For this review, take the finished solid that the model builds, in its own axes (mm). A direction names the side the tool comes from. Give positions to 0.01 mm unless a question says otherwise; leave off trailing zeros. Loops run counter-clockwise (first coordinate to the right, second up) from the corner with the lowest first, then second, coordinate; pieces in that order, holes last. Notation, with made-up numbers: (35, 2.5) - (57, 2.5) arc R20 ccw to (57, 15.5) - close; hole circle Ø8 at (19.5, 72.5). An arc over 180 degrees is marked (long way). Answer in a Markdown table with one row per item.
```python
from build123d import *

# Parameters (mm, degrees)
SKETCH_2_W          = 57
SKETCH_2_H          = 40.4
EXTRUDE_1_DEPTH     = 1.5
SKETCH_4_R          = 3
SKETCH_4_R_2        = 1.5
EXTRUDE_3_DEPTH     = 4
SKETCH_5_W          = 57
SKETCH_5_H          = 4.2
CUT_EXTRUDE_1_DEPTH = 2.5
SKETCH_6_W          = 1
SKETCH_6_H          = 32
EXTRUDE_4_DEPTH     = 1.5
SKETCH_8_R          = 3
SKETCH_8_R_2        = 1.5
CUT_EXTRUDE_3_DEPTH = 2
SKETCH_7_R          = 1.5
CUT_EXTRUDE_4_DEPTH = 4.5


with BuildPart() as part:
    # 草图2 → 凸台-拉伸1 (new body)
    with BuildSketch(Plane(origin=(0, 0, 0), x_dir=(1, 0, 0), z_dir=(0, 1, 0))):
        with Locations((3.861898857, -4.534326193)):
            Rectangle(SKETCH_2_W, SKETCH_2_H)
    extrude(amount=EXTRUDE_1_DEPTH)

    # 草图4 → 凸台-拉伸3 (add)
    with BuildSketch(Plane(origin=(0, 1.5, 0), x_dir=(1, 0, 0), z_dir=(0, 1, 0))):
        with Locations((-22.099370277, 7.765673807)):
            Circle(SKETCH_4_R)
        with Locations((-22.099370277, 7.765673807)):
            Circle(SKETCH_4_R_2, mode=Mode.SUBTRACT)
        with Locations((-22.138101143, -16.834326193)):
            Circle(SKETCH_4_R)
        with Locations((-22.138101143, -16.834326193)):
            Circle(SKETCH_4_R_2, mode=Mode.SUBTRACT)
        with Locations((29.861898857, -16.834326193)):
            Circle(SKETCH_4_R)
        with Locations((29.861898857, -16.834326193)):
            Circle(SKETCH_4_R_2, mode=Mode.SUBTRACT)
        with Locations((29.861898857, 7.765673807)):
            Circle(SKETCH_4_R)
        with Locations((29.861898857, 7.765673807)):
            Circle(SKETCH_4_R_2, mode=Mode.SUBTRACT)
    extrude(amount=EXTRUDE_3_DEPTH)

    # 草图5 → 切除-拉伸1 (cut, through all)
    with BuildSketch(Plane(origin=(0, 1.5, 0), x_dir=(1, 0, 0), z_dir=(0, 1, 0))):
        with Locations((3.861898857, 13.565673807)):
            Rectangle(SKETCH_5_W, SKETCH_5_H)
        with Locations((3.861898857, -22.634326193)):
            Rectangle(SKETCH_5_W, SKETCH_5_H)
    extrude(amount=-CUT_EXTRUDE_1_DEPTH, mode=Mode.SUBTRACT)

    # 草图6 → 凸台-拉伸4 (add)
    with BuildSketch(Plane(origin=(0, 1.5, 0), x_dir=(1, 0, 0), z_dir=(0, 1, 0))):
        with Locations((-25.138101143, -4.534326193)):
            Rectangle(SKETCH_6_W, SKETCH_6_H)
        with Locations((32.861898857, -4.534326193)):
            Rectangle(SKETCH_6_W, SKETCH_6_H)
    extrude(amount=-EXTRUDE_4_DEPTH)

    # 草图8 → 切除-拉伸3 (cut)
    with BuildSketch(Plane(origin=(0, 5.5, 0), x_dir=(1, 0, 0), z_dir=(0, 1, 0))):
        with Locations((-22.138101143, -16.834326193)):
            Circle(SKETCH_8_R)
        with Locations((29.861898857, -16.834326193)):
            Circle(SKETCH_8_R)
        with Locations((29.861898857, -16.834326193)):
            Circle(SKETCH_8_R_2, mode=Mode.SUBTRACT)
        with Locations((29.861898857, 7.765673807)):
            Circle(SKETCH_8_R)
        with Locations((29.861898857, 7.765673807)):
            Circle(SKETCH_8_R_2, mode=Mode.SUBTRACT)
        with Locations((-22.099370277, 7.765673807)):
            Circle(SKETCH_8_R)
        with Locations((-22.099370277, 7.765673807)):
            Circle(SKETCH_8_R_2, mode=Mode.SUBTRACT)
    extrude(amount=-CUT_EXTRUDE_3_DEPTH, mode=Mode.SUBTRACT)

    # 草图7 → 切除-拉伸4 (cut, through all)
    with BuildSketch(Plane.XZ):
        with Locations((29.861898857, 16.834326193)):
            Circle(SKETCH_7_R)
        with Locations((29.861898857, -7.765673807)):
            Circle(SKETCH_7_R)
        with Locations((-22.099370277, -7.765673807)):
            Circle(SKETCH_7_R)
        with Locations((-22.138101143, 16.834326193)):
            Circle(SKETCH_7_R)
    extrude(amount=-CUT_EXTRUDE_4_DEPTH, mode=Mode.SUBTRACT)


solid = part.part
```
1. We need section A-A, the plane y = 2.55. Give the boundary of the cut face in (x, z).
Values:
| item | result |
|---|---|
| outline | circle Ø6 at (-22.14, 16.83); circle Ø6 at (-22.1, -7.77); circle Ø6 at (29.86, -7.77); circle Ø6 at (29.86, 16.83); hole circle Ø3 at (-22.14, 16.83); hole circle Ø3 at (-22.1, -7.77); hole circle Ø3 at (29.86, -7.77); hole circle Ø3 at (29.86, 16.83) |
2. We need section B-B, the plane x = 25.5. Give the boundary of the cut face in (y, z), and give its area (3 significant figures).
Values:
| item | result |
|---|---|
| outline | (0, -11.47) - (1.5, -11.47) - (1.5, 20.53) - (0, 20.53) - close |
| area | 48.0 mm^2 |
3. Mouldability with a two-part tool opening along X and no side actions: class faces 1 (the face through (-25.638, 1, 5)), 2 (the face through (32.723, 2.486, 15.933)), 3 (the face through (-22.42, 1.73, -9.23)), 4 (the face through (3, 1, -11.466)) as released by +X, released by -X, zero draft, split by the parting line, or undercut.
Values:
| item | result |
|---|---|
| face 1 | released by -X |
| face 2 | undercut |
| face 3 | undercut |
| face 4 | zero draft |
4. For faces 5 (the face through (-23.637, 1.726, 16.9)), 6 (the face through (3, 1.5, 4)), list the 3-axis set-ups (+Z, -Z, +X, -X, +Y, -Y) from which the entire face can be reached by the end or side of a thin tool; tool diameter is ignored.
Values:
| item | result |
|---|---|
| face 5 | +Y, -Y |
| face 6 | +Y |
5. Wall thickness on line 1 (X direction, y = 1.95, z = 18); line 2 (Z direction, x = -21, y = 2.9); line 3 (Y direction, x = 22.5, z = 13): over which ranges is each line inside the solid? List them lowest first. Write a range as [from, to].
Values:
| item | result |
|---|---|
| line 1 | x = [-24.9, -23.08], [-21.19, -19.37], [27.1, 28.92], [30.81, 32.63] |
| line 2 | z = [-10.56, -8.79], [-6.75, -4.97], [14.06, 15.86], [17.81, 19.61] |
| line 3 | y = [0, 1.5] |
6. Clearance check with flat-ended pins moving along their axes: pin 1 (5 mm diameter, centred on x = 29.86, z = -7.77, fed in from +Y); pin 2 (2 mm diameter, centred on x = 6.5, z = 15, fed in from +Y); pin 3 (1.8 mm diameter, centred on x = 29.86, z = 16.83, fed in from +Y). State where each tip first meets the part, or that it passes through.
Values:
| item | result |
|---|---|
| pin 1 | stops at y = 3.5 |
| pin 2 | stops at y = 1.5 |
| pin 3 | passes through |
7. We need section C-C, the plane z = 11. Give the boundary of the cut face in (x, y).
Values:
| item | result |
|---|---|
| outline | (-25.64, 0) - (33.36, 0) - (33.36, 1.5) - (-25.64, 1.5) - close |
